Here's how the part is built. I have some questions about the finished solid (model axes, mm). Face numbers are marked on the shaded views. A direction names the side the tool comes from. Coordinates: 2 decimals unless noted, no trailing zeros. Loops run counter-clockwise (first coordinate to the right, second up) from the corner with the lowest first, then second, coordinate; pieces in that order, holes last.
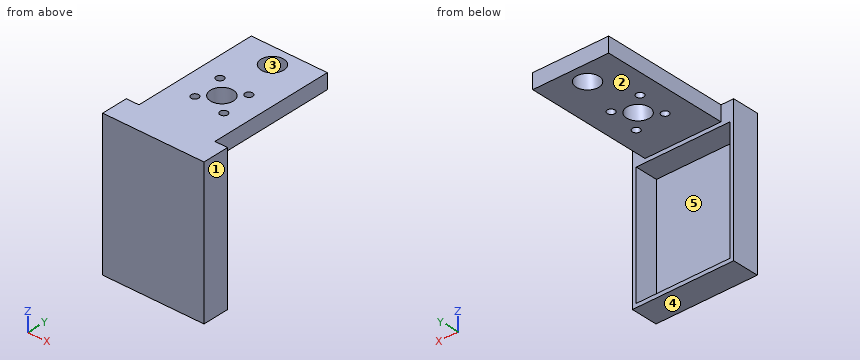
Autodesk Inventor part; units mm, degrees
ref_plane "YZ Plane" through (0, 0, 0) normal (1, 0, 0) x (0, 1, 0)
ref_plane "XZ Plane" through (0, 0, 0) normal (0, 1, 0) x (-1, 0, 0)
ref_plane "XY Plane" through (0, 0, 0) normal (0, 0, 1) x (1, 0, 0)
sketch "Sketch1" plane through (0, 0, 0) normal (0, 1, 0) x (-1, 0, 0)
  line L0 (18.5, -24) -> (-18.5, -24)
  line L1 (-18.5, -24) -> (-18.5, 24)
  line L2 (-18.5, 24) -> (18.5, 24)
  line L3 (18.5, 24) -> (18.5, -24)
  line L4 (20, -25.5) -> (-20, -25.5)
  line L5 (-20, -25.5) -> (-20, 25.5)
  line L6 (-20, 25.5) -> (20, 25.5)
  line L7 (20, 25.5) -> (20, -25.5)
  point P0 (0, 0)
  point P1 (0, -24)
  point P2 (-18.5, 0)
  point P3 (-20, 0)
  point P4 (0, -25.5)
  dimension "d0" = 37
  dimension "d1" = 48
  dimension "d2" = 1.5
  dimension "d3" = 1.5
extrude "Extrusion1" add sketch "Sketch1" along normal blind 9
extrude "Extrusion2" add sketch "Sketch1" against normal blind 1.5 contours L0 L1 L2 L3 | L4 L5 L6 L7
sketch "Sketch2" plane through (-20, 9, 25.5) normal (0, 0, 1) x (1, 0, 0)
  line L0 (5, 35) -> (35, 35) construction
  line L1 (35, 35) -> (35, 5)
  line L2 (35, 5) -> (5, 5) construction
  line L3 (5, 5) -> (5, 35)
  circle A0 centre (20, 20) radius 4.5
  circle A1 centre (14.3431, 14.3431) radius 1.5
  circle A2 centre (13.2825, 26.7175) radius 1.5
  circle A3 centre (25.6569, 25.6569) radius 1.5
  circle A4 centre (26.7175, 13.2825) radius 1.5
  line L4 (14.3431, 14.3431) -> (25.6569, 25.6569) construction
  line L5 (13.2825, 26.7175) -> (26.7175, 13.2825) construction
  line L6 (0, 0) -> (40, 0)
  line L7 (25.6569, 25.6569) -> (35, 35) construction
  line L8 (40, -10.5) -> (40, 0)
  line L9 (0, 0) -> (40, 0)
  line L10 (0, 0) -> (0, -10.5)
  line L11 (40, -10.5) -> (0, -10.5)
  circle A5 centre (20, 20) radius 13.9 construction
  line L12 (5, 5) -> (5, 0)
  line L13 (35, 5) -> (35, 0)
  circle A6 centre (20, 42.5) radius 4.5
  line L14 (5, 35) -> (5, 50)
  line L15 (5, 50) -> (35, 50)
  line L16 (35, 50) -> (35, 35)
  point P0 (20, -9)
  point P1 (20, 35)
  point P2 (35, 20)
  point P3 (20, 5)
  point P4 (20, 0)
  point P5 (5, 0)
  point P6 (35, 0)
  point P7 (5, 0)
  point P8 (35, 0)
  dimension "d8" = 9
  dimension "d9" = 3
  dimension "d10" = 16
  dimension "d11" = 19
  dimension "d12" = 30
  dimension "d16" = 27.8
  dimension "d17" = 5
  dimension "d19" = 7.5
  dimension "d20" = 15
extrude "Extrusion3" add sketch "Sketch2" along normal blind 6
equation "\"d20\" = 2 * d19"
properties part number "Motor Stand"
Q1. We'd pull the mould along X, two halves only. Please class the marked faces 1, 2 and 3: pulls with the +X half, pulls with the -X half, needs draft (parallel to the pull), parting line crosses it, or undercut.
Q2. For the marked faces 4 and 5, which set-ups out of +Z, -Z, +X, -X, +Y, -Y let a thin tool reach every point of the face, with its end or its side?
Q3. Suppose I cut it at C-C on z = 4.5. Write out the boundary of the cut face in (x, y), and give its area (3 significant figures).
Q4. Suppose I cut it at A-A on x = 0. Write out the boundary of the cut face in (y, z).
Q5. Suppose I cut it at D-D on x = 14. Write out the boundary of the cut face in (y, z), and give its area (4 significant figures).
Q6. Suppose I cut it at B-B on y = 51.5. Write out the boundary of the cut face in (x, z).
Q7. Please list where these lines run through material, in increasing order: probe 1 along Y at (x, z) = (0, 29); probe 2 along Z at (x, y) = (-2, 5.5); probe 3 along X at (y, z) = (2, 23.5).
Q8. Will these pins go through, and if not, where does the flat tip stop? P1, Ø20, axis at x = -5.5, z = -1.5, coming from the +Y side; P2, Ø8, axis at x = 0, y = 29, coming from the -Z side; P3, Ø1.8, axis at y = 33, z = 28, coming from the +X side; P4, Ø3.5, axis at x = 5.66, y = 34.66, coming from the -Z side.
Check values:
1. face 1: pulls with the +X half
1. face 2: needs draft
1. face 3: undercut
2. face 4: -Z, +X, -X, +Y, -Y
2. face 5: +Y
3. outline: (-20, -1.5) - (20, -1.5) - (20, 9) - (18.5, 9) - (18.5, 0) - (-18.5, 0) - (-18.5, 9) - (-20, 9) - close
3. area: 87.0 mm2
4. outline: (-1.5, -25.5) - (9, -25.5) - (9, -24) - (0, -24) - (0, 24) - (9, 24) - (9, 25.5) - (24.5, 25.5) - (24.5, 31.5) - (-1.5, 31.5) - close; (33.5, 25.5) - (47, 25.5) - (47, 31.5) - (33.5, 31.5) - close; (56, 25.5) - (59, 25.5) - (59, 31.5) - (56, 31.5) - close
5. outline: (-1.5, -25.5) - (9, -25.5) - (9, -24) - (0, -24) - (0, 24) - (9, 24) - (9, 25.5) - (59, 25.5) - (59, 31.5) - (-1.5, 31.5) - close
5. area: 466.5 mm2
6. outline: (-15, 25.5) - (-4.5, 25.5) - (-4.5, 31.5) - (-15, 31.5) - close; (4.5, 25.5) - (15, 25.5) - (15, 31.5) - (4.5, 31.5) - close
7. probe 1: y = -1.5 to 24.5, 33.5 to 47, 56 to 59
7. probe 2: z = -25.5 to -24, 24 to 31.5
7. probe 3: x = -20 to -18.5, 18.5 to 20
8. P1: stops at y = 0
8. P2: passes through
8. P3: stops at x = 15
8. P4: stops at z = 25.5
